```python
from build123d import *

# Parameters (mm, degrees)
SKETCH_1_W          = 25
SKETCH_1_H          = 23
EXTRUDE_1_DEPTH     = 12
CUT_EXTRUDE_START   = 1
SKETCH_2_W          = 25
SKETCH_2_H          = 21
CUT_EXTRUDE_1_DEPTH = 11
EXTRUDE_START       = 12
SKETCH_6_W          = 25
SKETCH_6_H          = 23
EXTRUDE_3_DEPTH     = 1
CUT_EXTRUDE_START_2 = 13
SKETCH_8_R          = 9.75
CUT_EXTRUDE_2_DEPTH = 1
SKETCH_9_W          = 25
SKETCH_9_H          = 23
CUT_EXTRUDE_3_DEPTH = 1


with BuildPart() as part:
    # 스케치1 → 보스-돌출1 (new body)
    with BuildSketch(Plane(origin=(0, 0, 0), x_dir=(1, 0, 0), z_dir=(0, 1, 0))):
        Rectangle(SKETCH_1_W, SKETCH_1_H)
    extrude(amount=EXTRUDE_1_DEPTH)

    # 스케치2 → 컷-돌출1 (cut)
    with BuildSketch(Plane(origin=(0, 0, 0), x_dir=(1, 0, 0), z_dir=(0, 1, 0)).offset(CUT_EXTRUDE_START)):
        with Locations((1, 0)):
            Rectangle(SKETCH_2_W, SKETCH_2_H)
    extrude(amount=CUT_EXTRUDE_1_DEPTH, mode=Mode.SUBTRACT)


with BuildPart() as body_2:
    # 스케치6 → 보스-돌출3 (new body)
    with BuildSketch(Plane(origin=(0, 0, 0), x_dir=(1, 0, 0), z_dir=(0, 1, 0)).offset(EXTRUDE_START)):
        Rectangle(SKETCH_6_W, SKETCH_6_H)
    extrude(amount=EXTRUDE_3_DEPTH)

    # 스케치8 → 컷-돌출2 (cut)
    with BuildSketch(Plane(origin=(0, 0, 0), x_dir=(1, 0, 0), z_dir=(0, 1, 0)).offset(CUT_EXTRUDE_START_2)):
        with Locations(Location((-0.75, 0, 0), (0, 0, 270))):
            Circle(SKETCH_8_R)
    extrude(amount=-CUT_EXTRUDE_2_DEPTH, mode=Mode.SUBTRACT)

    # 스케치9 → 컷-돌출3 (cut)
    with BuildSketch(Plane(origin=(0, 13, 0), x_dir=(1, 0, 0), z_dir=(0, 1, 0))):
        Rectangle(SKETCH_9_W, SKETCH_9_H)
    extrude(amount=-CUT_EXTRUDE_3_DEPTH, mode=Mode.SUBTRACT)


solid = part.part
```
Geometry check sheet. Reference: the model listing, model coordinates, mm. A direction names the side the tool comes from. Give positions to 0.01 mm unless a question says otherwise; leave off trailing zeros. Order: outer loops, then holes, each group sorted by start corner. A loop starts at its lowest first (then second) coordinate and runs counter-clockwise, first axis right, second up. Notation, with made-up numbers: (31.25, 77.5) -> (68.25, 77.5) arc R27 cw to (68.25, 112.5) -> close; hole circle Ø2 at (-36.5, -19.75). An arc over 180 degrees is marked (long way). Write each question's results on one line, items separated by ' | '. Start each with the question number.
(1) Access from +Z, -Z, +X, -X, +Y, -Y to the whole of each face (thin tool, end or side, straight path). Record for faces 4 (the face through (0, 6, 11.5)), 5 (the face through (-11.5, 6, 0)).
(2) Sectioned sample at B-B (y = 3.75). Enter the section's corners in (x, z).
(3) Scan lines: line 1 (Z direction, x = 10.25, y = 5.5); line 2 (Y direction, x = -3.75, z = 2); line 3 (X direction, y = 8.25, z = -9.5). Record each from-to range of solid material in increasing order.
(4) Sectioned sample at C-C (z = -2.5). Enter the section's corners in (x, y), plus the area to 3 significant figures.
(5) Mould release check, pull along Z, two halves, no side actions. Record for faces 1 (the face through (12.5, 0.6, 0.9)), 2 (the face through (0, 6, -10.5)), 3 (the face through (0, 6, -11.5)): pulls with the +Z half, pulls with the -Z half, needs draft (parallel to the pull), parting line crosses it, or undercut.
(6) Gauge pin test, flat end, axial feed: P1, Ø6.5, axis at x = 2.5, z = -3.5, coming from the +Y side. Record the tip position at first contact, or that the pin passes through.
(7) Sectioned sample at A-A (x = -3.25). Enter the section's corners in (y, z), plus the area to 3 significant figures.
Answer below:
1) face 4: +Z, +X, -X, +Y, -Y | face 5: +X, +Y
2) outline: (-12.5, -11.5) -> (12.5, -11.5) -> (12.5, -10.5) -> (-11.5, -10.5) -> (-11.5, 10.5) -> (12.5, 10.5) -> (12.5, 11.5) -> (-12.5, 11.5) -> close
3) line 1: -11.5 to -10.5, 10.5 to 11.5 | line 2: 0 to 1 | line 3: -12.5 to -11.5
4) outline: (-12.5, 0) -> (12.5, 0) -> (12.5, 1) -> (-11.5, 1) -> (-11.5, 12) -> (-12.5, 12) -> close | area: 36.0 mm2
5) face 1: needs draft | face 2: undercut | face 3: pulls with the -Z half
6) P1: y = 1
7) outline: (0, -11.5) -> (12, -11.5) -> (12, -10.5) -> (1, -10.5) -> (1, 10.5) -> (12, 10.5) -> (12, 11.5) -> (0, 11.5) -> close | area: 45.0 mm2
